Geometry: final body of the model. Coordinates: model frame, mm. Face numbers are marked on the shaded views. Round coordinates to 2 decimals unless told otherwise and drop trailing zeros. Order: outer loops, then holes, each group sorted by start corner. A loop starts at its lowest first (then second) coordinate and runs counter-clockwise, first axis right, second up. Notation, with made-up numbers: (66, 89) - (110, 89) arc R12 cw to (110, 104) - close; hole circle Ø8 at (80.5, 79). An arc over 180 degrees is marked (long way). Put each result on its own line as item: value. Start each with the question number.
(1) Section A-A (x = 7.5). Output: boundary loops of the cut face in (y, z), and give its area (3 significant figures).
(2) Pull-direction query (Z, two-part tool) for the marked faces 1, 2 and 3; classes: released by +Z, released by -Z, zero draft, split by the parting line, or undercut.
(3) Material intervals for L1, parallel to Y at x = 9.75, z = 0; L2, parallel to Y at x = 28.8, z = 0; L3, parallel to X at y = 7.25, z = -6, sorted ascending. Write a range as [from, to].
(4) Pin query (flat end, axial travel): P1, Ø8.5, axis at y = -2, z = 0, coming from the +X side; P2, Ø3, axis at x = 9.5, z = 6, coming from the -Y side; P3, Ø2, axis at x = 3.5, y = 2.5, coming from the +Z side; P4, Ø1.5, axis at y = 6.5, z = 4.5, coming from the +X side. Return the tip coordinate at first contact, or that it passes through.
from build123d import *

# Parameters (mm, degrees)
CHAMFER1_SIZE = 0.2


with BuildPart() as part:
    # Sketch1 → Revolve1 (revolve)
    with BuildSketch(Plane.XY, mode=Mode.PRIVATE) as revolve1_sk:
        Polygon((0.5, 5), (0.5, 8.5), (0, 8.5), (0, 9.5), (3.5, 9.5), (3.5, 9), (4.8, 9), (4.8, 9.5), (24.2, 9.5), (24.2, 9), (25.5, 9), (25.5, 9.5), (29, 9.5), (29, 8.5), (28.5, 8.5), (28.5, 5), align=None)
    revolve(revolve1_sk.sketch.rotate(Axis((0, 0, 0), (1, 0, 0)), 90), axis=Axis((0, 0, 0), (1, 0, 0)))

    # Chamfer1
    chamfer1_edges = [part.edges().sort_by_distance(p)[0] for p in [
        (29, 0, -9.5),
        (0, 0, -9.5),
    ]]
    chamfer(chamfer1_edges, length=CHAMFER1_SIZE)


solid = part.part
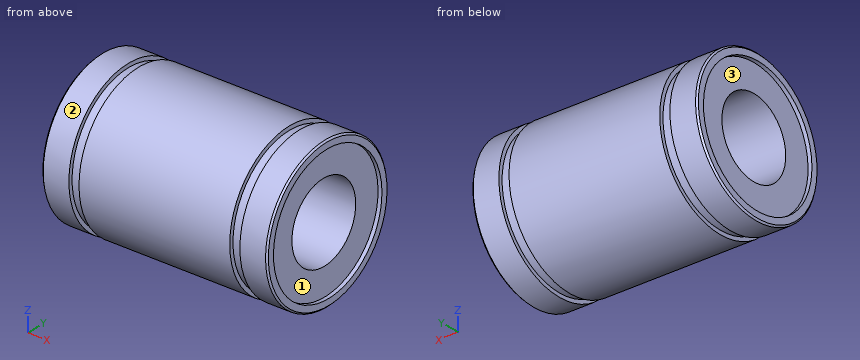
Checks:
1. outline: circle Ø19 at (0, 0); hole circle Ø10 at (0, 0)
1. area: 205 mm²
2. face 1: undercut
2. face 2: split by the parting line
2. face 3: undercut
3. L1: y = [-9.5, -5], [5, 9.5]
3. L2: y = [-9.5, -8.5], [8.5, 9.5]
3. L3: x = [0.11, 3.5], [4.8, 24.2], [25.5, 28.89]
4. P1: stops at x = 28.5
4. P2: stops at y = -8.37
4. P3: stops at z = 9.38
4. P4: stops at x = 29
